```python
from build123d import *

# Parameters (mm, degrees)
SKETCH1_R           = 1.143
BOSS_EXTRUDE1_DEPTH = 2.7


with BuildPart() as part:
    # Sketch1 → Boss-Extrude1 (new body)
    with BuildSketch(Plane(origin=(0, 0, 0), x_dir=(1, 0, 0), z_dir=(0, 1, 0))):
        with BuildLine():
            Line((-11.327327395, -33.908852397), (-11.327327395, -50.658852397))
            Line((-11.327327395, -50.658852397), (-10.311327339, -50.658852397))
            ThreePointArc((-10.311327339, -50.658852397), (15.050108966, -26.657976598), (-7.517327395, -0.012990077))
            Line((-7.517327395, -0.012990077), (-11.327327395, -0.012990077))
            Line((-11.327327395, -0.012990077), (-11.327327395, -19.407100798))
            Line((-11.327327395, -19.407100798), (-31.421327339, -19.407100798))
            Line((-31.421327339, -19.407100798), (-31.421327339, -33.908852397))
            Line((-31.421327339, -33.908852397), (-11.327327395, -33.908852397))
        make_face()
        with Locations(Location((-7.517327395, -16.497976598, 0), (0, 0, 90))):
            Circle(SKETCH1_R, mode=Mode.SUBTRACT)
        with Locations(Location((-7.517327395, -36.817976598, 0), (0, 0, 90))):
            Circle(SKETCH1_R, mode=Mode.SUBTRACT)
        with Locations(Location((5.182672605, -26.657976598, 0), (0, 0, 90))):
            Circle(SKETCH1_R, mode=Mode.SUBTRACT)
    extrude(amount=BOSS_EXTRUDE1_DEPTH)


solid = part.part
```
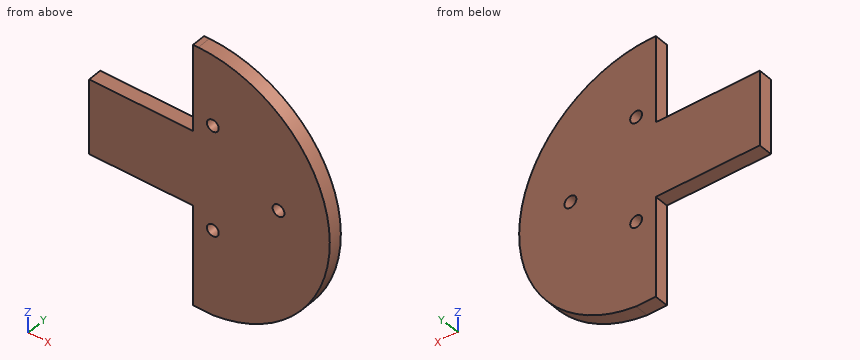
Here's how the part is built. I have some questions about the finished solid (model axes, mm). Give positions to 0.01 mm unless a question says otherwise; leave off trailing zeros. Loops run counter-clockwise (first coordinate to the right, second up) from the corner with the lowest first, then second, coordinate; pieces in that order, holes last. Notation, with made-up numbers: (67, 25.25) -> (93, 25.25) arc R23 cw to (93, 47.25) -> close; hole circle Ø6 at (64, 51). An arc over 180 degrees is marked (long way). Use one line per item in the form item = value. Start each with the question number.
1) Please list where these lines run through material, in increasing order: line 1 along Z through (x, y) = (-12, 1.8); line 2 along X through (y, z) = (1.95, 37.5); line 3 along Z through (x, y) = (3.5, 2.3).
2) Imagine slicing it at A-A (y = 1.7). Please give me the cut outline in (x, z).
3) Imagine slicing it at B-B (x = -20). Please give me the cut outline in (y, z), then the cut area to 3 significant figures.
4) Imagine slicing it at C-C (z = 45). Please give me the cut outline in (x, y).
5) For P1, Ø1.4, axis at x = -22.5, y = 1.5, coming from the +Z side; P2, Ø1.4, axis at x = -23, y = 1, coming from the -Z side; P3, Ø1.4, axis at y = 1, z = 12, coming from the -X side, each with a flat end and sliding along its axis, tell me the tip position at first contact or that it passes through.
Check values:
q1.line_1 = 19.41 to 33.91
q1.line_2 = -11.33 to -8.43, -6.6 to 11.94
q1.line_3 = 3.94 to 46.58
q2.outline = (-31.42, 19.41) -> (-11.33, 19.41) -> (-11.33, 0.01) -> (-7.52, 0.01) arc R25.4 ccw to (-10.31, 50.66) -> (-11.33, 50.66) -> (-11.33, 33.91) -> (-31.42, 33.91) -> close; hole circle Ø2.29 at (-7.52, 16.5); hole circle Ø2.29 at (-7.52, 36.82); hole circle Ø2.29 at (5.18, 26.66)
q3.outline = (0, 19.41) -> (2.7, 19.41) -> (2.7, 33.91) -> (0, 33.91) -> close
q3.area = 39.2 mm^2
q4.outline = (-11.33, 0) -> (5.67, 0) -> (5.67, 2.7) -> (-11.33, 2.7) -> close
q5.P1 = 33.91
q5.P2 = 19.41
q5.P3 = -11.33
